The listing builds one solid part. Answer for the finished solid, in the listing's coordinates (mm). Coordinates: 2 decimals unless noted, no trailing zeros. Order: outer loops, then holes, each group sorted by start corner. A loop starts at its lowest first (then second) coordinate and runs counter-clockwise, first axis right, second up. Notation, with made-up numbers: (10, 8) -> (58, 8) arc R25 ccw to (58, 42) -> close; hole circle Ø11 at (43, 88.5). An arc over 180 degrees is marked (long way). Put each result on its own line as item: value. Start each with the question number.
```python
from build123d import *

# Parameters (mm, degrees)
SKETCH_1_R      = 4
EXTRUDE_1_DEPTH = 5


with BuildPart() as part:
    # 草图1 → 凸台-拉伸1 (new body)
    with BuildSketch(Plane(origin=(0, 0, 0), x_dir=(1, 0, 0), z_dir=(0, 1, 0))):
        Polygon((3.205904539, 6.141838169), (-3.716035611, 5.847313857), (-6.921940149, -0.294524312), (-3.205904539, -6.141838169), (3.716035611, -5.847313857), (6.921940149, 0.294524312), align=None)
        with Locations(Location((0, 0, 0), (0, 0, 270))):
            Circle(SKETCH_1_R, mode=Mode.SUBTRACT)
    extrude(amount=EXTRUDE_1_DEPTH)

    # 草图2 → 切除-旋转1 (revolve, cut)
    with BuildSketch(Plane(origin=(0, 0, 0), x_dir=(0.4627324620846592, 0, -0.8864979799937897), z_dir=(0.8864979799937897, 0, 0.4627324620846592)), mode=Mode.PRIVATE) as cut_revolve_1_sk:
        Polygon((-6.92820323, 4.5), (-6.92820323, 5), (-5.92820323, 5), align=None)
        Polygon((-6.92820323, 0.5), (-6.92820323, 0), (-5.92820323, 0), align=None)
    revolve(cut_revolve_1_sk.sketch.rotate(Axis((0, 0, 0), (0, 1, 0)), 207.563569327), axis=Axis((0, 0, 0), (0, 1, 0)), mode=Mode.SUBTRACT)


solid = part.part
```
(1) Find the intervals of material crossed by L1, parallel to Z at x = -1.5, y = 1.6; L2, parallel to X at y = 0.5, z = 1; L3, parallel to Z at x = 1.25, y = 1.3, in increasing order.
(2) Each of these flat-tipped pins is pushed along its axis until it touches: P1, Ø1, axis at x = -4.5, y = 0.5, coming from the -Z side; P2, Ø2, axis at x = 2, y = 4, coming from the -Z side; P3, Ø4, axis at x = -3, z = -4.5, coming from the -Y side; P4, Ø1.5, axis at y = 1, z = 1.5, coming from the +X side. Where does it stop, or does it pass through?
(3) The part is cut by section A-A on z = 0. Determine the outline of the cut face in (x, y).
(4) The part is cut by section B-B on y = 1.5. Determine the outline of the cut face in (x, z), plus the area to 3 significant figures.
Worked out:
1. L1: -5.94 to -3.71, 3.71 to 6.07
1. L2: -6.47 to -3.87, 3.87 to 6.25
1. L3: -6.06 to -3.8, 3.8 to 5.95
2. P1: z = -5.3
2. P2: z = -6.13
2. P3: y = 0
2. P4: x = 6.38
3. outline: (-6.77, 0.42) -> (-5.93, 0) -> (-4, 0) -> (-4, 5) -> (-5.93, 5) -> (-6.77, 4.58) -> close; (4, 0) -> (5.93, 0) -> (6.77, 0.42) -> (6.77, 4.58) -> (5.93, 5) -> (4, 5) -> close
4. outline: (-6.92, 0.29) -> (-3.72, -5.85) -> (3.21, -6.14) -> (6.92, -0.29) -> (3.72, 5.85) -> (-3.21, 6.14) -> close; hole circle Ø8 at (0, 0)
4. area: 74.4 mm2
